Could you check a few things on this model? Use its own coordinates, in mm. A direction names the side the tool comes from. Coordinates: 2 decimals unless noted, no trailing zeros. Loops run counter-clockwise (first coordinate to the right, second up) from the corner with the lowest first, then second, coordinate; pieces in that order, holes last. Notation, with made-up numbers: (87.5, -29) - (130.5, -29) arc R24 cw to (130.5, 10) - close; hole circle Ø3 at (62.5, 38). An arc over 180 degrees is marked (long way). Use CSV: the item, a comma, the result in double quotes.
from build123d import *

# Parameters (mm, degrees)
SKETCH3_W           = 30
SKETCH3_H           = 15
BOSS_EXTRUDE1_DEPTH = 10
SKETCH4_W           = 20
SKETCH4_H           = 7
CUT_EXTRUDE1_DEPTH  = 16
SKETCH5_R           = 1.5
CUT_EXTRUDE2_DEPTH  = 5


with BuildPart() as part:
    # Sketch3 → Boss-Extrude1 (new body)
    with BuildSketch(Plane(origin=(0, 0, 0), x_dir=(1, 0, 0), z_dir=(0, 1, 0))):
        Rectangle(SKETCH3_W, SKETCH3_H)
    extrude(amount=BOSS_EXTRUDE1_DEPTH)

    # Sketch4 → Cut-Extrude1 (cut, through all)
    with BuildSketch(Plane.XY.offset(7.5)):
        with Locations((0, 3.5)):
            Rectangle(SKETCH4_W, SKETCH4_H)
    extrude(amount=-CUT_EXTRUDE1_DEPTH, mode=Mode.SUBTRACT)

    # Sketch5 → Cut-Extrude2 (cut)
    with BuildSketch(Plane.XZ):
        with Locations((12.5, 0)):
            Circle(SKETCH5_R)
        with Locations((-12.5, 0)):
            Circle(SKETCH5_R)
    extrude(amount=-CUT_EXTRUDE2_DEPTH, mode=Mode.SUBTRACT)


solid = part.part
(1) Thinking about a two-plate mould opening in X: for faces 4 (the face through (11, 2, 0)), 5 (the face through (-15, 5, 0)), 6 (the face through (-0.2, 7.2, 7.5)), which applies, +X half, -X half, draft (parallel to the pull), parting line (faces both ways), or undercut?
Computed:
face 4,"undercut"
face 5,"-X half"
face 6,"draft"
(2) Suppose I cut it at D-D (z = 0.5). Write out the boundary of the cut face in (x, y).
Computed:
outline,"(-15, 0) - (-13.91, 0) - (-13.91, 5) - (-11.09, 5) - (-11.09, 0) - (-10, 0) - (-10, 7) - (10, 7) - (10, 0) - (11.09, 0) - (11.09, 5) - (13.91, 5) - (13.91, 0) - (15, 0) - (15, 10) - (-15, 10) - close"
(3) Suppose I cut it at B-B (z = -5.25). Write out the boundary of the cut face in (x, y), plus the area to 3 significant figures.
Computed:
outline,"(-15, 0) - (-10, 0) - (-10, 7) - (10, 7) - (10, 0) - (15, 0) - (15, 10) - (-15, 10) - close"
area,"160 mm²"
(4) Which directions (+Z, -Z, +X, -X, +Y, -Y) give clear straight access to the entire face, cutting with the end or side of a thin tool? Please do faces 1 (the face through (-13, 5, 0)), 2 (the face through (10, 3, 0)), 3 (the face through (-0.2, 7.2, -7.5)).
Computed:
face 1,"-Y"
face 2,"+Z, -Z, -Y"
face 3,"-Z, +X, -X, +Y, -Y"
(5) Suppose I cut it at C-C (x = 12.5). Write out the boundary of the cut face in (y, z), plus the area to 3 significant figures.
Computed:
outline,"(0, -7.5) - (10, -7.5) - (10, 7.5) - (0, 7.5) - (0, 1.5) - (5, 1.5) - (5, -1.5) - (0, -1.5) - close"
area,"135 mm²"
(6) Will these pins go through, and if not, where does the flat tip stop? pin 1 (1.8 mm diameter, centred on x = 12.5, z = 0, fed in from -Y); pin 2 (1.5 mm diameter, centred on x = 6.5, z = -4.5, fed in from -Y).
Computed:
pin 1,"stops at y = 5"
pin 2,"stops at y = 7"
(7) Suppose I cut it at A-A (y = 1.25). Write out the boundary of the cut face in (x, z), plus the area to 3 significant figures.
Computed:
outline,"(-15, -7.5) - (-10, -7.5) - (-10, 7.5) - (-15, 7.5) - close; (10, -7.5) - (15, -7.5) - (15, 7.5) - (10, 7.5) - close; hole circle Ø3 at (-12.5, 0); hole circle Ø3 at (12.5, 0)"
area,"136 mm²"
(8) Please list where these lines run through material, in increasing order: line 1 (X direction, y = 6, z = 1); line 2 (Z direction, x = 12.5, y = 1.25); line 3 (Y direction, x = -5.25, z = -3.75).
Computed:
line 1,"x = -15 to -10, 10 to 15"
line 2,"z = -7.5 to -1.5, 1.5 to 7.5"
line 3,"y = 7 to 10"
